Here's how the part is built. I have some questions about the finished solid (model axes, mm). Face numbers are marked on the shaded views. A direction names the side the tool comes from. Give positions to 0.01 mm unless a question says otherwise; leave off trailing zeros. Order: outer loops, then holes, each group sorted by start corner. A loop starts at its lowest first (then second) coordinate and runs counter-clockwise, first axis right, second up. Notation, with made-up numbers: (45.25, -8.5) - (66.25, -8.5) arc R31 ccw to (66.25, 20.5) - close; hole circle Ø1 at (47.5, 71). An arc over 180 degrees is marked (long way). One line per question, with ' | ' between items.
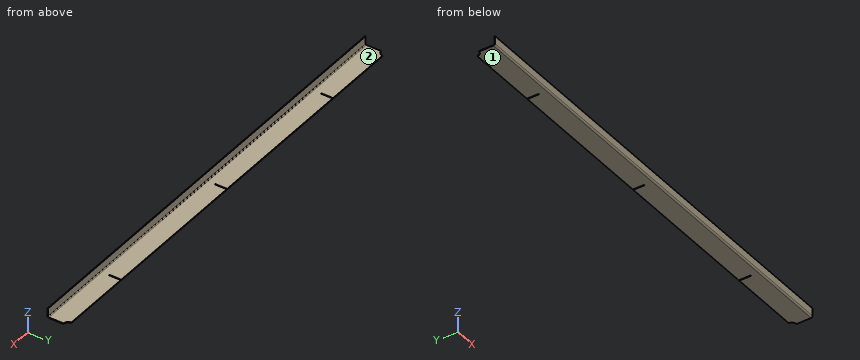
Autodesk Inventor part; units mm, degrees
ref_plane "YZ Plane" through (0, 0, 0) normal (1, 0, 0) x (0, 1, 0)
ref_plane "XZ Plane" through (0, 0, 0) normal (0, 1, 0) x (-1, 0, 0)
ref_plane "XY Plane" through (0, 0, 0) normal (0, 0, 1) x (1, 0, 0)
sketch "Sketch1" plane through (0, 0, 0) normal (0, 0, 1) x (1, 0, 0)
  line L0 (-750, 67.4521) -> (750, 67.4521)
  line L1 (750, 67.4521) -> (750, 0)
  line L2 (750, 0) -> (-750, 0)
  line L3 (-750, 0) -> (-750, 67.4521)
  point P0 (0, 0)
  point P1 (0, 0)
  dimension "d0" = 1500
  dimension "d1" = 67.4521
extrude "Plate1" add sketch "Sketch1" along normal blind 2
sketch "Sketch2" plane through (750, 2, 0) normal (0, -1, 0) x (1, 0, 0)
  line L0 (-1500, 0) -> (0, 0)
  line L1 (0, 0) -> (0, 30)
  line L2 (0, 30) -> (-1500, 30)
  line L3 (-1500, 30) -> (-1500, 0)
edge flange "Flange1" height 30 angle 90 thickness 2 bend radius 2.75 thickness toward (0, -1, 0) relief round relief width 2 relief depth 1 edges at (0, 0, 2) wall of the first edge with corners at (-750, 2, 0) (750, 2, 0) (750, 2, 30) (-750, 2, 30)
bend "Bend1"
corner "Corner1"
sketch "Sketch5" plane through (0, 0, 0) normal (0, 0, -1) x (-1, 0, 0)
  line L0 (750, 67.4521) -> (-750, 67.4521)
  line L1 (499, 67.4521) -> (499, 29)
  line L2 (499, 29) -> (501, 29)
  line L3 (501, 29) -> (501, 67.4521)
  line L4 (750, 0) -> (-750, 0)
  point P0 (0, 0)
  point P1 (500, 29)
  dimension "d18" = 2
  dimension "d20" = 29
  dimension "d27" = 250
extrude "Extrusion1" cut sketch "Sketch5" against normal through all
pattern_linear "Rectangular Pattern1" count 3 spacing 500 along (1, 0, 0) of "Extrusion1"
sketch "Sketch6" plane through (0, 0, 0) normal (0, 0, -1) x (-1, 0, 0)
  line L0 (-750, 67.4521) -> (-750, 4.75)
  circle A0 centre (-750, 67.4521) radius 15
  line L1 (-750, 67.4521) -> (-501, 67.4521)
  point P0 (0, 0)
  point P1 (-735, 67.4521)
  point P2 (-750, 52.4521)
  dimension "d24" = 30
extrude "Extrusion2" cut sketch "Sketch6" against normal through all contours L1 A0 L0 picked at (-740.1254, 66.3395)
mirror "Mirror1" about plane through (0, 0, 0) normal (1, 0, 0) of "Extrusion2"
equation "\"d1\" = Стрингер_2"
equation "\"d18\" = Thickness"
equation "\"d2\" = Thickness"
equation "\"d3\" = BendReliefWidth"
equation "\"d4\" = BendReliefDepth"
equation "\"d5\" = MinimumRemnant"
equation "\"d6\" = TransitionRadius"
equation "\"d9\" = BendRadius"
equation "\"d10\" = CornerReliefSize"
equation "\"d11\" = GapSize"
equation "\"d12\" = JacobiRadiusSize"
equation "\"GapSize\" = Thickness"
equation "\"MinimumRemnant\" = 2 * Thickness"
equation "\"BendReliefDepth\" = 0.5 * Thickness"
equation "\"BendReliefWidth\" = Thickness"
equation "\"CornerReliefSize\" = 4 * Thickness"
equation "\"JacobiRadiusSize\" = BendRadius"
equation "\"TransitionRadius\" = BendRadius"
equation "\"qqqqqq\" = 67.35706"
properties part number "МОО 052 стрингер спина 2" material "Stainless Steel"
1) On a 3-axis mill with a long thin cutter (end or side, diameter ignored), from which of +Z, -Z, +X, -X, +Y, -Y can I reach the whole of each face in a straight line? I mean the marked faces 1 and 2. Say none if no direction works.
Model answer:
face 1: -Z, +X, -X, +Y, -Y | face 2: +Z, +X, -X, +Y
2) I want a section at B-B (z = 20.5). List the corners of the cut face in (x, y) for me, plus the area to 3 significant figures.
Model answer:
outline: (-750, 0) - (750, 0) - (750, 2) - (-750, 2) - close | area: 3,000 mm2
3) I'm going to push flat-ended pins straight in: P1, Ø1, axis at y = 57.5, z = 0.5, coming from the -X side; P2, Ø0.6, axis at y = 54, z = 1, coming from the -X side; P3, Ø8, axis at x = 156, y = 11, coming from the -Z side; P4, Ø6, axis at x = -397.5, z = 13.5, coming from the +Y side. Where does each tip first touch, or does it pass through?
Model answer:
P1: stops at x = -739.24 | P2: stops at x = -744.01 | P3: stops at z = 0 | P4: stops at y = 2
4) Please list where these lines run through material, in increasing order: L1, parallel to Z at x = 324.5, y = 33.5; L2, parallel to Y at x = -67.5, z = 1.75.
Model answer:
L1: z = 0 to 2 | L2: y = 1.07 to 67.45
5) I want a section at A-A (x = -482). List the corners of the cut face in (y, z) for me, plus the area to 3 significant figures.
Model answer:
outline: (0, 4.75) arc R4.75 ccw to (4.75, 0) - (67.45, 0) - (67.45, 2) - (4.75, 2) arc R2.75 cw to (2, 4.75) - (2, 30) - (0, 30) - close | area: 188 mm2
